CAD build for the part. Positions are in the model's coordinates, mm. A direction names the side the tool comes from. Coordinates: 2 decimals unless noted, no trailing zeros. Order: outer loops, then holes, each group sorted by start corner. A loop starts at its lowest first (then second) coordinate and runs counter-clockwise, first axis right, second up. Notation, with made-up numbers: M -27,52.5 L -4,52.5 A25 cw -4,89.5 Z; hole C 19.5,89 d7. An arc over 180 degrees is marked long. Write item = value, one per line.
from build123d import *

# Parameters (mm, degrees)
F0_R     = 12.7
F1_DEPTH = 35
F2_W     = 34.810588
F2_H     = 34.74434
F3_DEPTH = 5


with BuildPart() as f1:
    # F0 (on Right) → F1 (new body)
    with BuildSketch(Plane.YZ):
        Circle(F0_R)
    extrude(amount=F1_DEPTH)

    # F2 (on face) → F3 (join)
    with BuildSketch(Plane.YZ.offset(35)):
        Rectangle(F2_W, F2_H)
    extrude(amount=F3_DEPTH)

    # F4 (on face) → F5 (revolve, cut)
    with BuildSketch(Plane(origin=(0, 0, 0), x_dir=(0, -1, 0), z_dir=(-1, 0, 0))):
        with BuildLine():
            ThreePointArc((0, 38.1), (-25.4, 12.7), (0, -12.7))
            Line((0, -12.7), (0, 38.1))
        make_face()
    revolve(axis=Axis((0, 0, 12.7), (0, 0, 1)), mode=Mode.SUBTRACT)


solid = f1.part
(1) Slice it at B-B, the plane z = 0. Write the cut outline in (x, y).
Evaluation:
outline = M 17.96,-12.7 L 35,-12.7 L 35,-17.41 L 40,-17.41 L 40,17.41 L 35,17.41 L 35,12.7 L 17.96,12.7 A22 cw Z
(2) Tool access for faces 1 (the face through (40, 0, 0)), 2 (the face through (35, 7, 12)): list every direction of +Z, -Z, +X, -X, +Y, -Y with a clear straight run to the whole face (end or side of a thin tool).
Evaluation:
face_1 = +Z, -Z, +X, +Y, -Y
face_2 = -X
(3) Slice it at A-A, the plane y = 0. Write the cut outline in (x, z), then the cut area to 3 significant figures.
Evaluation:
outline = M 0,-12.7 L 35,-12.7 L 35,-17.37 L 40,-17.37 L 40,17.37 L 35,17.37 L 35,12.7 L 25.4,12.7 A25.4 cw Z
area = 556 mm²
(4) Slice it at C-C, the plane x = 29. Write the cut outline in (y, z), then the cut area to 3 significant figures.
Evaluation:
outline = C 0,0 d25.4
area = 507 mm²
(5) Slice it at D-D, the plane y = 14.5. Write the cut outline in (x, z), then the cut area to 3 significant figures.
Evaluation:
outline = M 35,-17.37 L 40,-17.37 L 40,17.37 L 35,17.37 Z
area = 174 mm²
(6) Pin check, flat tips, straight feed: pin 1 Ø1.5 at (x, y) = (25.5, 0.5) entering from +Z; pin 2 Ø6 at (x, z) = (29, 13) entering from -Y; pin 3 Ø8 at (x, y) = (9.5, -1) entering from -Z. Stop position of each tip, or through.
Evaluation:
pin_1 = 12.7
pin_2 = -7.83
pin_3 = -12.7
(7) Wall check: line 1 (X direction, y = -5, z = 15); line 2 (Y direction, x = 33, z = 4); line 3 (Z direction, x = 15.5, y = -10). Give the ranges that are in metal, low to high. Write a range as from..to.
Evaluation:
line_1 = 35..40
line_2 = -12.05..12.05
line_3 = -7.83..-4.76
